Model file for the job. Use its own axes, mm. Face numbers are marked on the shaded views. Give positions to 0.01 mm unless a question says otherwise; leave off trailing zeros. Write each loop counter-clockwise with the first axis right and the second up, starting at its lowest first coordinate (ties: lowest second). Pieces come first, ordered by that corner, then holes.
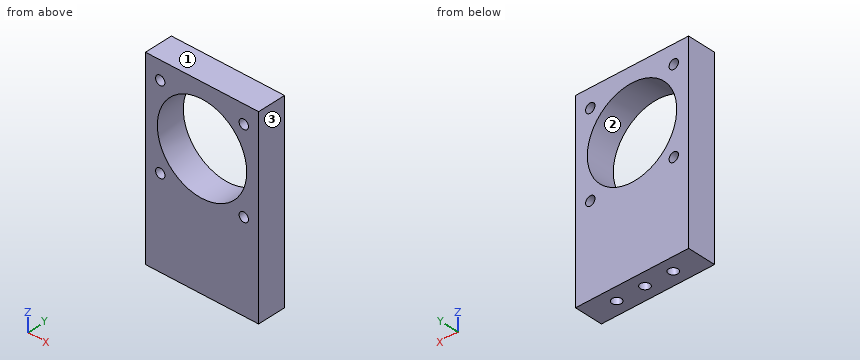
```python
from build123d import *

# Parameters (mm, degrees)
F0_W     = 101.6
F0_H     = 171.45
F1_DEPTH = 25.4
F3_D     = 8.4328
F3_DEPTH = 25.4
F3_TIP   = 2.5334687141
F4_R     = 40.132
F5_DEPTH = 25.401
F7_D     = 8.4


with BuildPart() as f1:
    # F0 (on Front) → F1 (new body)
    with BuildSketch(Plane.XZ):
        Rectangle(F0_W, F0_H)
    extrude(amount=F1_DEPTH)

    # F3
    with Locations(Plane(origin=(0, 0, -85.725), x_dir=(1, 0, 0), z_dir=(0, 0, -1))):
        with Locations((-25.4, 12.7), (25.4, 12.7), (0, 12.7)):
            Hole(F3_D / 2, depth=F3_DEPTH)
            with Locations((0, 0, -(F3_DEPTH + F3_TIP / 2))):  # 118° drill point
                Cone(0, F3_D / 2, F3_TIP, mode=Mode.SUBTRACT)

    # F4 (on face) → F5 (cut, through all)
    with BuildSketch(Plane.XZ.offset(25.4)):
        with Locations((0, 31.75)):
            Circle(F4_R)
    extrude(amount=-F5_DEPTH, mode=Mode.SUBTRACT)

    # F7 (through all)
    with Locations(Plane.XZ.offset(25.4)):
        with Locations((-37.4904, 69.2404), (37.4904, 69.2404), (37.4904, -5.7404), (-37.4904, -5.7404)):
            Hole(F7_D / 2)


solid = f1.part
```
1. Pin check, flat tip, straight feed: P1, Ø5, axis at x = 0, y = -12.7, coming from the -Z side. Stop position of the tip, or through.
Calculated:
P1: stops at z = -59.29
2. Slice it at C-C, the plane y = -6.5. Write the cut outline in (x, z) (3 decimals).
Calculated:
outline: (-50.8, -85.725) - (50.8, -85.725) - (50.8, 85.725) - (-50.8, 85.725) - close; hole circle Ø8.4 at (-37.49, -5.74); hole circle Ø8.4 at (-37.49, 69.24); hole circle Ø80.264 at (0, 31.75); hole circle Ø8.4 at (37.49, -5.74); hole circle Ø8.4 at (37.49, 69.24)
3. Pull direction X, two halves, no side cores. Call the marked faces 1, 2 and 3: +X half, -X half, draft (parallel to the pull), parting line (faces both ways), or undercut.
Calculated:
face 1: draft
face 2: undercut
face 3: +X half
4. Slice it at B-B, the plane x = -10. Write the cut outline in (y, z) (3 decimals), and give its area (3 significant figures).
Calculated:
outline: (-25.4, -85.725) - (0, -85.725) - (0, -7.116) - (-25.4, -7.116) - close; (-25.4, 70.616) - (0, 70.616) - (0, 85.725) - (-25.4, 85.725) - close
area: 2,380 mm2
5. Probe probe 1 along X at (y, z) = (-4.5, 66.5); probe 2 along Y at (x, z) = (-25.4, -65.5); probe 3 along Z at (x, y) = (-1.5, -3) (3 decimals). List the from-to ranges inside material, lowest first.
Calculated:
probe 1: x = -50.8 to -40.67, -34.31 to -20.08, 20.08 to 34.31, 40.67 to 50.8
probe 2: y = -25.4 to -16.92, -8.48 to 0
probe 3: z = -85.725 to -8.354, 71.854 to 85.725
6. Slice it at D-D, the plane x = 36. Write the cut outline in (y, z) (3 decimals).
Calculated:
outline: (-25.4, -85.725) - (0, -85.725) - (0, -9.667) - (-25.4, -9.667) - close; (-25.4, -1.814) - (0, -1.814) - (0, 14.014) - (-25.4, 14.014) - close; (-25.4, 49.486) - (0, 49.486) - (0, 65.314) - (-25.4, 65.314) - close; (-25.4, 73.167) - (0, 73.167) - (0, 85.725) - (-25.4, 85.725) - close
7. Slice it at A-A, the plane z = 31.75. Write the cut outline in (x, y).
Calculated:
outline: (-50.8, -25.4) - (-40.13, -25.4) - (-40.13, 0) - (-50.8, 0) - close; (40.13, -25.4) - (50.8, -25.4) - (50.8, 0) - (40.13, 0) - close
